```python
from build123d import *
from OCP.BRepFilletAPI import BRepFilletAPI_MakeChamfer

# Parameters (mm, degrees)
SKETCH_1_W               = 7.5
SKETCH_1_H               = 5.8
EXTRUDE_1_DEPTH          = 7
CUT_EXTRUDE_1_DEPTH      = 9.454140997
CUT_EXTRUDE_1_DEPTH_BACK = 9.454140997
SKETCH_2_W               = 1.7
SKETCH_2_H               = 0.2
SKETCH_3_W               = 5.9
SKETCH_3_H               = 4.2
CUT_EXTRUDE_2_DEPTH      = 6.2
CUT_EXTRUDE_3_DEPTH      = 1
CUT_EXTRUDE_4_DEPTH      = 9.454140997
CUT_EXTRUDE_4_DEPTH_BACK = 9.454140997
SKETCH_5_W               = 1
SKETCH_5_H               = 3.4
SKETCH_6_W               = 0.6
SKETCH_6_H               = 0.6
EXTRUDE_3_DEPTH          = 4.2
SKETCH_7_W               = 0.6
SKETCH_7_H               = 0.6
EXTRUDE_4_DEPTH          = 3.5
CHAMFER_1_SIZE           = 0.3
CHAMFER_1_SIZE2          = 0.10919107


with BuildPart() as part:
    # 草图1 → 凸台-拉伸1 (new body)
    with BuildSketch(Plane(origin=(0, 0, 0), x_dir=(1, 0, 0), z_dir=(0, 1, 0))):
        Rectangle(SKETCH_1_W, SKETCH_1_H)
    extrude(amount=EXTRUDE_1_DEPTH)

    # 草图2 → 切除-拉伸1 (cut, two sides: drawn at the far end of the back side and taken through both)
    with BuildSketch(Plane.XY.offset(-CUT_EXTRUDE_1_DEPTH_BACK)):
        with Locations((-1.4, 0.1)):
            Rectangle(SKETCH_2_W, SKETCH_2_H)
        with Locations((1.4, 0.1)):
            Rectangle(SKETCH_2_W, SKETCH_2_H)
    extrude(amount=CUT_EXTRUDE_1_DEPTH + CUT_EXTRUDE_1_DEPTH_BACK, mode=Mode.SUBTRACT)

    # 草图3 → 切除-拉伸2 (cut)
    with BuildSketch(Plane(origin=(0, 7, 0), x_dir=(1, 0, 0), z_dir=(0, 1, 0))):
        Rectangle(SKETCH_3_W, SKETCH_3_H)
    extrude(amount=-CUT_EXTRUDE_2_DEPTH, mode=Mode.SUBTRACT)

    # 草图4 → 切除-拉伸3 (cut)
    with BuildSketch(Plane.XY.offset(2.9)):
        Polygon((-1.95, 7), (-1.55, 6.6), (-1.95, 5.907179677), (-1.95, 3.2), (1.95, 3.2), (1.95, 5.907179677), (1.55, 6.6), (1.95, 7), align=None)
    extrude(amount=-CUT_EXTRUDE_3_DEPTH, mode=Mode.SUBTRACT)

    # 草图5 → 切除-拉伸4 (cut, two sides: drawn at the far end of the back side and taken through both)
    with BuildSketch(Plane.ZY.offset(-CUT_EXTRUDE_4_DEPTH_BACK)):
        with Locations((1.6, 5.3)):
            Rectangle(SKETCH_5_W, SKETCH_5_H)
    extrude(amount=CUT_EXTRUDE_4_DEPTH + CUT_EXTRUDE_4_DEPTH_BACK, mode=Mode.SUBTRACT)

    # 草图6 → 凸台-拉伸3 (add)
    with BuildSketch(Plane.XZ.offset(-0.2)):
        with Locations((-1.27, 0.4)):
            Rectangle(SKETCH_6_W, SKETCH_6_H)
        with Locations((1.27, 0.4)):
            Rectangle(SKETCH_6_W, SKETCH_6_H)
    extrude(amount=EXTRUDE_3_DEPTH)

    # 草图7 → 凸台-拉伸4 (add)
    with BuildSketch(Plane(origin=(0, 0.8, 0), x_dir=(1, 0, 0), z_dir=(0, 1, 0))):
        with Locations((1.27, -0.4)):
            Rectangle(SKETCH_7_W, SKETCH_7_H)
        with Locations((-1.27, -0.4)):
            Rectangle(SKETCH_7_W, SKETCH_7_H)
    extrude(amount=EXTRUDE_4_DEPTH)

    # 倒角1: one chamfer whose edges measure the first distance from different faces: ONE call of the kernel's chamfer builder (chamfer() names one face for all edges)
    chamfer_1_edges_1 = [part.edges().sort_by_distance(p)[0] for p in [
        (-1.27, -4, 0.7),
    ]]
    chamfer_1_side_1 = [part.faces().sort_by_distance(p)[0] for p in [
        (-1.27, -1.9, 0.7),
    ]]
    chamfer_1_edges_2 = [part.edges().sort_by_distance(p)[0] for p in [
        (-1.57, -4, 0.4),
    ]]
    chamfer_1_side_2 = [part.faces().sort_by_distance(p)[0] for p in [
        (-1.57, -1.9, 0.4),
    ]]
    chamfer_1_edges_3 = [part.edges().sort_by_distance(p)[0] for p in [
        (-1.27, -4, 0.1),
    ]]
    chamfer_1_side_3 = [part.faces().sort_by_distance(p)[0] for p in [
        (-1.27, -1.9, 0.1),
    ]]
    chamfer_1_edges_4 = [part.edges().sort_by_distance(p)[0] for p in [
        (-0.97, -4, 0.4),
    ]]
    chamfer_1_side_4 = [part.faces().sort_by_distance(p)[0] for p in [
        (-0.97, -1.9, 0.4),
    ]]
    chamfer_1_edges_5 = [part.edges().sort_by_distance(p)[0] for p in [
        (1.27, -4, 0.1),
    ]]
    chamfer_1_side_5 = [part.faces().sort_by_distance(p)[0] for p in [
        (1.27, -1.9, 0.1),
    ]]
    chamfer_1_edges_6 = [part.edges().sort_by_distance(p)[0] for p in [
        (1.57, -4, 0.4),
    ]]
    chamfer_1_side_6 = [part.faces().sort_by_distance(p)[0] for p in [
        (1.57, -1.9, 0.4),
    ]]
    chamfer_1_edges_7 = [part.edges().sort_by_distance(p)[0] for p in [
        (1.27, -4, 0.7),
    ]]
    chamfer_1_side_7 = [part.faces().sort_by_distance(p)[0] for p in [
        (1.27, -1.9, 0.7),
    ]]
    chamfer_1_edges_8 = [part.edges().sort_by_distance(p)[0] for p in [
        (0.97, -4, 0.4),
    ]]
    chamfer_1_side_8 = [part.faces().sort_by_distance(p)[0] for p in [
        (0.97, -1.9, 0.4),
    ]]
    chamfer_1_edges_9 = [part.edges().sort_by_distance(p)[0] for p in [
        (1.27, 4.3, 0.7),
    ]]
    chamfer_1_side_9 = [part.faces().sort_by_distance(p)[0] for p in [
        (1.27, 2.55, 0.7),
    ]]
    chamfer_1_edges_10 = [part.edges().sort_by_distance(p)[0] for p in [
        (1.57, 4.3, 0.4),
    ]]
    chamfer_1_side_10 = [part.faces().sort_by_distance(p)[0] for p in [
        (1.57, 2.55, 0.4),
    ]]
    chamfer_1_edges_11 = [part.edges().sort_by_distance(p)[0] for p in [
        (1.27, 4.3, 0.1),
    ]]
    chamfer_1_side_11 = [part.faces().sort_by_distance(p)[0] for p in [
        (1.27, 2.55, 0.1),
    ]]
    chamfer_1_edges_12 = [part.edges().sort_by_distance(p)[0] for p in [
        (0.97, 4.3, 0.4),
    ]]
    chamfer_1_side_12 = [part.faces().sort_by_distance(p)[0] for p in [
        (0.97, 2.55, 0.4),
    ]]
    chamfer_1_edges_13 = [part.edges().sort_by_distance(p)[0] for p in [
        (-1.57, 4.3, 0.4),
    ]]
    chamfer_1_side_13 = [part.faces().sort_by_distance(p)[0] for p in [
        (-1.57, 2.55, 0.4),
    ]]
    chamfer_1_edges_14 = [part.edges().sort_by_distance(p)[0] for p in [
        (-1.27, 4.3, 0.7),
    ]]
    chamfer_1_side_14 = [part.faces().sort_by_distance(p)[0] for p in [
        (-1.27, 2.55, 0.7),
    ]]
    chamfer_1_edges_15 = [part.edges().sort_by_distance(p)[0] for p in [
        (-0.97, 4.3, 0.4),
    ]]
    chamfer_1_side_15 = [part.faces().sort_by_distance(p)[0] for p in [
        (-0.97, 2.55, 0.4),
    ]]
    chamfer_1_edges_16 = [part.edges().sort_by_distance(p)[0] for p in [
        (-1.27, 4.3, 0.1),
    ]]
    chamfer_1_side_16 = [part.faces().sort_by_distance(p)[0] for p in [
        (-1.27, 2.55, 0.1),
    ]]
    chamfer_1 = BRepFilletAPI_MakeChamfer(part.part.solid().wrapped)
    for e in chamfer_1_edges_1:
        chamfer_1.Add(CHAMFER_1_SIZE, CHAMFER_1_SIZE2, e.wrapped, chamfer_1_side_1[0].wrapped)  # the first distance lies on this face
    for e in chamfer_1_edges_2:
        chamfer_1.Add(CHAMFER_1_SIZE, CHAMFER_1_SIZE2, e.wrapped, chamfer_1_side_2[0].wrapped)  # the first distance lies on this face
    for e in chamfer_1_edges_3:
        chamfer_1.Add(CHAMFER_1_SIZE, CHAMFER_1_SIZE2, e.wrapped, chamfer_1_side_3[0].wrapped)  # the first distance lies on this face
    for e in chamfer_1_edges_4:
        chamfer_1.Add(CHAMFER_1_SIZE, CHAMFER_1_SIZE2, e.wrapped, chamfer_1_side_4[0].wrapped)  # the first distance lies on this face
    for e in chamfer_1_edges_5:
        chamfer_1.Add(CHAMFER_1_SIZE, CHAMFER_1_SIZE2, e.wrapped, chamfer_1_side_5[0].wrapped)  # the first distance lies on this face
    for e in chamfer_1_edges_6:
        chamfer_1.Add(CHAMFER_1_SIZE, CHAMFER_1_SIZE2, e.wrapped, chamfer_1_side_6[0].wrapped)  # the first distance lies on this face
    for e in chamfer_1_edges_7:
        chamfer_1.Add(CHAMFER_1_SIZE, CHAMFER_1_SIZE2, e.wrapped, chamfer_1_side_7[0].wrapped)  # the first distance lies on this face
    for e in chamfer_1_edges_8:
        chamfer_1.Add(CHAMFER_1_SIZE, CHAMFER_1_SIZE2, e.wrapped, chamfer_1_side_8[0].wrapped)  # the first distance lies on this face
    for e in chamfer_1_edges_9:
        chamfer_1.Add(CHAMFER_1_SIZE, CHAMFER_1_SIZE2, e.wrapped, chamfer_1_side_9[0].wrapped)  # the first distance lies on this face
    for e in chamfer_1_edges_10:
        chamfer_1.Add(CHAMFER_1_SIZE, CHAMFER_1_SIZE2, e.wrapped, chamfer_1_side_10[0].wrapped)  # the first distance lies on this face
    for e in chamfer_1_edges_11:
        chamfer_1.Add(CHAMFER_1_SIZE, CHAMFER_1_SIZE2, e.wrapped, chamfer_1_side_11[0].wrapped)  # the first distance lies on this face
    for e in chamfer_1_edges_12:
        chamfer_1.Add(CHAMFER_1_SIZE, CHAMFER_1_SIZE2, e.wrapped, chamfer_1_side_12[0].wrapped)  # the first distance lies on this face
    for e in chamfer_1_edges_13:
        chamfer_1.Add(CHAMFER_1_SIZE, CHAMFER_1_SIZE2, e.wrapped, chamfer_1_side_13[0].wrapped)  # the first distance lies on this face
    for e in chamfer_1_edges_14:
        chamfer_1.Add(CHAMFER_1_SIZE, CHAMFER_1_SIZE2, e.wrapped, chamfer_1_side_14[0].wrapped)  # the first distance lies on this face
    for e in chamfer_1_edges_15:
        chamfer_1.Add(CHAMFER_1_SIZE, CHAMFER_1_SIZE2, e.wrapped, chamfer_1_side_15[0].wrapped)  # the first distance lies on this face
    for e in chamfer_1_edges_16:
        chamfer_1.Add(CHAMFER_1_SIZE, CHAMFER_1_SIZE2, e.wrapped, chamfer_1_side_16[0].wrapped)  # the first distance lies on this face
    add(Compound.cast(chamfer_1.Shape()), mode=Mode.REPLACE)


solid = part.part
```
Verification items for the finished model (mm, model axes). A direction names the side the tool comes from. Round coordinates to 2 decimals unless told otherwise and drop trailing zeros. Order: outer loops, then holes, each group sorted by start corner. A loop starts at its lowest first (then second) coordinate and runs counter-clockwise, first axis right, second up. Notation, with made-up numbers: (78, -38) -> (98, -38) arc R19 cw to (98, -2) -> close; hole circle Ø2 at (-25, 1). An arc over 180 degrees is marked (long way). Put each result on its own line as item: value. Start each with the question number.
(1) Depth check by flat-ended pin: pin 1 Ø1.2 at (x, z) = (3, -0.5) entering from -Y; pin 2 Ø0.7 at (y, z) = (-1, 0.5) entering from -X; pin 3 Ø2 at (x, y) = (0.5, -2) entering from +Z. Enter the tip coordinate at first touch or a pass-through.
(2) Tool access check on faces 4 (the face through (-2.95, 4, 0)), 5 (the face through (-0.1, 7, -2.3)), 6 (the face through (-3.3, 5.3, 1.1)). Record the directions out of +Z, -Z, +X, -X, +Y, -Y that give a thin tool (end or side, any length) a straight path to the whole face; none if there is none.
(3) Section check B-B (y = 6.75). Enter the section's corners in (x, z), then the cut area to 3 significant figures.
(4) Section check C-C (z = -2.45). Enter the section's corners in (x, y).
(5) Draft check along X on faces 1 (the face through (0, 3, 2.1)), 2 (the face through (-3.3, 3.6, 1.6)), 3 (the face through (-3.75, 3, 0)). Enter one of: +X half, -X half, draft (parallel to the pull), parting line (faces both ways), or undercut.
(6) Section check D-D (y = 3.75). Enter the section's corners in (x, z), then the cut area to 3 significant figures.
(7) Section check A-A (y = 2.25). Enter the section's corners in (x, z), then the cut area to 3 significant figures.
(8) Material ranges on line 1 along Z through (x, y) = (-1.25, 2); line 2 along X through (y, z) = (4.5, 2.7); line 3 along X through (y, z) = (1.5, 1.45), recorded low to high.
Completed:
1. pin 1: stops at y = 0
1. pin 2: stops at x = -1.57
1. pin 3: stops at z = 0.7
2. face 4: +Y
2. face 5: +Z, -Z, +X, -X, +Y
2. face 6: +X, -X, +Y
3. outline: (-3.75, -2.9) -> (3.75, -2.9) -> (3.75, 1.1) -> (2.95, 1.1) -> (2.95, -2.1) -> (-2.95, -2.1) -> (-2.95, 1.1) -> (-3.75, 1.1) -> close; (-3.75, 2.1) -> (-1.7, 2.1) -> (-1.7, 2.9) -> (-3.75, 2.9) -> close; (1.7, 2.1) -> (3.75, 2.1) -> (3.75, 2.9) -> (1.7, 2.9) -> close
3. area: 14.4 mm2
4. outline: (-3.75, 0) -> (-2.25, 0) -> (-2.25, 0.2) -> (-0.55, 0.2) -> (-0.55, 0) -> (0.55, 0) -> (0.55, 0.2) -> (2.25, 0.2) -> (2.25, 0) -> (3.75, 0) -> (3.75, 7) -> (-3.75, 7) -> close
5. face 1: undercut
5. face 2: draft
5. face 3: -X half
6. outline: (-3.75, -2.9) -> (3.75, -2.9) -> (3.75, 1.1) -> (2.95, 1.1) -> (2.95, -2.1) -> (-2.95, -2.1) -> (-2.95, 1.1) -> (-3.75, 1.1) -> close; (-3.75, 2.1) -> (-1.95, 2.1) -> (-1.95, 2.9) -> (-3.75, 2.9) -> close; (-1.57, 0.1) -> (-0.97, 0.1) -> (-0.97, 0.7) -> (-1.57, 0.7) -> close; (0.97, 0.1) -> (1.57, 0.1) -> (1.57, 0.7) -> (0.97, 0.7) -> close; (1.95, 2.1) -> (3.75, 2.1) -> (3.75, 2.9) -> (1.95, 2.9) -> close
6. area: 14.7 mm2
7. outline: (-3.75, -2.9) -> (3.75, -2.9) -> (3.75, 2.9) -> (-3.75, 2.9) -> close; (-1.57, 0.1) -> (-0.97, 0.1) -> (-0.97, 0.7) -> (-1.57, 0.7) -> close; (0.97, 0.1) -> (1.57, 0.1) -> (1.57, 0.7) -> (0.97, 0.7) -> close; hole (-2.95, -2.1) -> (2.95, -2.1) -> (2.95, 2.1) -> (-2.95, 2.1) -> close
7. area: 19.4 mm2
8. line 1: z = -2.9 to -2.1, 0.1 to 0.7, 2.1 to 2.9
8. line 2: x = -3.75 to -1.95, 1.95 to 3.75
8. line 3: x = -3.75 to -2.95, 2.95 to 3.75
